```python
from build123d import *

# Parameters (mm, degrees)
SKETCH3_R                       = 10
CUT_EXTRUDE1_DEPTH              = 104.923048473
F_6_0MM_DOWEL_HOLE1_D           = 6
F_6_0MM_DOWEL_HOLE1_CSINK_D     = 6.05
F_6_0MM_DOWEL_HOLE1_CSINK_ANGLE = 90


with BuildPart() as part:
    # Sketch2 → Revolve1 (revolve)
    with BuildSketch(Plane.XY, mode=Mode.PRIVATE) as revolve1_sk:
        with BuildLine():
            Line((4, 0), (4, 30))
            Line((4, 30), (0, 30))
            Line((0, 30), (0, 100))
            Line((0, 100), (10, 100))
            ThreePointArc((10, 100), (17.071067812, 97.071067812), (20, 90))
            Line((20, 90), (20, 26.294228634))
            Line((20, 26.294228634), (11.5, 17.794228634))
            Line((11.5, 17.794228634), (11.5, 7.794228634))
            Line((11.5, 7.794228634), (16, 0))
            Line((16, 0), (4, 0))
        make_face()
    revolve(revolve1_sk.sketch.rotate(Axis((0, 30, 0), (0, 1, 0)), 90), axis=Axis((0, 30, 0), (0, 1, 0)))

    # Sketch3 → Cut-Extrude1 (cut, through all)
    with BuildSketch(Plane.XZ):
        with Locations((0, 27)):
            Circle(SKETCH3_R)
        with Locations((27, 0)):
            Circle(SKETCH3_R)
        with Locations((0, -27)):
            Circle(SKETCH3_R)
        with Locations((-27, 0)):
            Circle(SKETCH3_R)
    extrude(amount=-CUT_EXTRUDE1_DEPTH, mode=Mode.SUBTRACT)

    # Ø6.0mm Dowel Hole1 (through all)
    with Locations(Plane(origin=(0.030615993, 12.647260725, 11.499959246), x_dir=(0.999996456179, 0, -0.002662260256), z_dir=(0.002662260256, 0, 0.999996456179))):
        with Locations((0, 0)):
            CounterSinkHole(F_6_0MM_DOWEL_HOLE1_D / 2, F_6_0MM_DOWEL_HOLE1_CSINK_D / 2, counter_sink_angle=F_6_0MM_DOWEL_HOLE1_CSINK_ANGLE)


solid = part.part
```
The model under review builds one solid part; all positions refer to its coordinate system, in mm. A direction names the side the tool comes from. Coordinates: 2 decimals unless noted, no trailing zeros. Write each loop counter-clockwise with the first axis right and the second up, starting at its lowest first coordinate (ties: lowest second). Pieces come first, ordered by that corner, then holes. Notation, with made-up numbers: (-24.5, -27.5) - (-2.5, -27.5) arc R19 cw to (-2.5, 8.5) - close; hole circle Ø8 at (47.5, 6.25). An arc over 180 degrees is marked (long way). Answer in a Markdown table with one row per item. Add a question column.
Q1. Consider section A-A on y = 43. Give the boundary of the cut face in (x, z).
Q2. To check wall thickness, follow line 1 along X through (y, z) = (16, 0); line 2 along X through (y, z) = (55, 0); line 3 along Y through (x, z) = (3, -14). State the ranges of each line that lie inside material, in increasing order. Write a range as from..to.
Q3. Consider section B-B on z = 0. Give the boundary of the cut face in (x, y), then the cut area to 3 significant figures.
Q4. Clearance check with flat-ended pins moving along their axes: pin 1 (1.5 mm diameter, centred on x = 12, y = 54.5, fed in from -Z); pin 2 (2 mm diameter, centred on y = 59.5, z = 13, fed in from -X); pin 3 (2.5 mm diameter, centred on x = 1.5, z = -2, fed in from -Y). State where each tip first meets the part, or that it passes through.
Q5. For faces 4 (the face through (0, 100, 0)), 5 (the face through (2.4, 15.2, 3.2)), 6 (the face through (11.5, 7.31, 2.55)), list the 3-axis set-ups (+Z, -Z, +X, -X, +Y, -Y) from which the entire face can be reached by the end or side of a thin tool; tool diameter is ignored.
Q6. Consider section C-C on y = 91. Give the boundary of the cut face in (x, z).
Q7. Draft analysis for pull direction Z (two halves, no side actions). For faces 1 (the face through (-3.45, 12.72, -10.97)), 2 (the face through (-17, 60, 0)), 3 (the face through (3, 0, -3)), state which applies: +Z half, -Z half, draft (parallel to the pull), parting line (faces both ways), or undercut.
Answers below:
| question | item | result |
|---|---|---|
| 1 | outline | (-19.06, -6.07) arc R20 ccw to (-6.07, -19.06) arc R10 cw to (6.07, -19.06) arc R20 ccw to (19.06, -6.07) arc R10 cw to (19.06, 6.07) arc R20 ccw to (6.07, 19.06) arc R10 cw to (-6.07, 19.06) arc R20 ccw to (-19.06, 6.07) arc R10 cw to start |
| 2 | line 1 | -11.5..-4, 4..11.5 |
| 2 | line 2 | -17..17 |
| 2 | line 3 | 0..2.91, 20.61..99.02 |
| 3 | outline | (-17, 23.29) - (-11.5, 17.79) - (-11.5, 7.79) - (-16, 0) - (-4, 0) - (-4, 30) - (4, 30) - (4, 0) - (16, 0) - (11.5, 7.79) - (11.5, 17.79) - (17, 23.29) - (17, 97.14) arc R10 ccw to (10, 100) - (-10, 100) arc R10 ccw to (-17, 97.14) - close |
| 3 | area | 2,960 mm² |
| 4 | pin 1 | z = -16.54 |
| 4 | pin 2 | x = -16 |
| 4 | pin 3 | y = 30 |
| 5 | face 4 | +Z, -Z, +X, -X, +Y |
| 5 | face 5 | -Y |
| 5 | face 6 | none |
| 6 | outline | (-19.02, -6.02) arc R19.95 ccw to (-6.02, -19.02) arc R10 cw to (6.02, -19.02) arc R19.95 ccw to (19.02, -6.02) arc R10 cw to (19.02, 6.02) arc R19.95 ccw to (6.02, 19.02) arc R10 cw to (-6.02, 19.02) arc R19.95 ccw to (-19.02, 6.02) arc R10 cw to start |
| 7 | face 1 | parting line |
| 7 | face 2 | undercut |
| 7 | face 3 | draft |
